from build123d import *

# Parameters (mm, degrees)
ESQUISSE1_R        = 6.75
ESQUISSE1_R_2      = 172
BOSS_EXTRU_1_DEPTH = 10


with BuildPart() as part:
    # Esquisse1 → Boss.-Extru.1 (new body)
    with BuildSketch(Plane.XY):
        with BuildLine():
            Line((220, -35), (220, -297.575677416))
            Line((220, -297.575677416), (190, -380))
            Line((190, -380), (165, -380))
            Line((165, -380), (165, -180))
            Line((165, -180), (125, -180))
            Line((125, -180), (125, -330))
            Line((125, -330), (-125, -330))
            Line((-125, -330), (-125, -180))
            Line((-125, -180), (-165, -180))
            Line((-165, -180), (-165, -380))
            Line((-165, -380), (-190, -380))
            Line((-190, -380), (-220, -297.575677416))
            Line((-220, -297.575677416), (-220, -35))
            Line((-220, -35), (-240, -35))
            Line((-240, -35), (-250, -25))
            Line((-250, -25), (-250, -20))
            Line((-250, -20), (-210, -20))
            Line((-210, -20), (-210, 20))
            Line((-210, 20), (-250, 20))
            Line((-250, 20), (-250, 25))
            Line((-250, 25), (-240, 35))
            Line((-240, 35), (-217.19806629, 35))
            ThreePointArc((-217.19806629, 35), (-155.563491861, 155.563491861), (-35, 217.19806629))
            Line((-35, 217.19806629), (-35, 240))
            Line((-35, 240), (-25, 250))
            Line((-25, 250), (-20, 250))
            Line((-20, 250), (-20, 210))
            Line((-20, 210), (20, 210))
            Line((20, 210), (20, 250))
            Line((20, 250), (25, 250))
            Line((25, 250), (35, 240))
            Line((35, 240), (35, 217.19806629))
            ThreePointArc((35, 217.19806629), (155.563491861, 155.563491861), (217.19806629, 35))
            Line((217.19806629, 35), (240, 35))
            Line((240, 35), (250, 25))
            Line((250, 25), (250, 20))
            Line((250, 20), (210, 20))
            Line((210, 20), (210, -20))
            Line((210, -20), (250, -20))
            Line((250, -20), (250, -25))
            Line((250, -25), (240, -35))
            Line((240, -35), (220, -35))
        make_face()
        with Locations((0, 195)):
            Circle(ESQUISSE1_R, mode=Mode.SUBTRACT)
        Circle(ESQUISSE1_R_2, mode=Mode.SUBTRACT)
        with Locations((52.610370376, 187.768871033)):
            Circle(ESQUISSE1_R, mode=Mode.SUBTRACT)
        with Locations((101.318870257, 166.611783887)):
            Circle(ESQUISSE1_R, mode=Mode.SUBTRACT)
        with Locations((142.513013034, 133.097862928)):
            Circle(ESQUISSE1_R, mode=Mode.SUBTRACT)
        with Locations((173.137617588, 89.712682358)):
            Circle(ESQUISSE1_R, mode=Mode.SUBTRACT)
        with Locations((190.921397098, 39.673922545)):
            Circle(ESQUISSE1_R, mode=Mode.SUBTRACT)
        with Locations((194.545409992, -13.307270606)):
            Circle(ESQUISSE1_R, mode=Mode.SUBTRACT)
        with Locations((183.740879813, -65.301524373)):
            Circle(ESQUISSE1_R, mode=Mode.SUBTRACT)
        with Locations((159.309129137, -112.452662812)):
            Circle(ESQUISSE1_R, mode=Mode.SUBTRACT)
        with Locations((123.062149144, -151.263701687)):
            Circle(ESQUISSE1_R, mode=Mode.SUBTRACT)
        with Locations((77.68821252, -178.856203794)):
            Circle(ESQUISSE1_R, mode=Mode.SUBTRACT)
        with Locations((26.552496574, -193.183759477)):
            Circle(ESQUISSE1_R, mode=Mode.SUBTRACT)
        with Locations((-26.552496574, -193.183759477)):
            Circle(ESQUISSE1_R, mode=Mode.SUBTRACT)
        with Locations((-77.68821252, -178.856203794)):
            Circle(ESQUISSE1_R, mode=Mode.SUBTRACT)
        with Locations((-123.062149144, -151.263701687)):
            Circle(ESQUISSE1_R, mode=Mode.SUBTRACT)
        with Locations((-159.309129137, -112.452662812)):
            Circle(ESQUISSE1_R, mode=Mode.SUBTRACT)
        with Locations((-183.740879813, -65.301524373)):
            Circle(ESQUISSE1_R, mode=Mode.SUBTRACT)
        with Locations((-194.545409992, -13.307270606)):
            Circle(ESQUISSE1_R, mode=Mode.SUBTRACT)
        with Locations((-190.921397098, 39.673922545)):
            Circle(ESQUISSE1_R, mode=Mode.SUBTRACT)
        with Locations((-173.137617588, 89.712682358)):
            Circle(ESQUISSE1_R, mode=Mode.SUBTRACT)
        with Locations((-142.513013034, 133.097862928)):
            Circle(ESQUISSE1_R, mode=Mode.SUBTRACT)
        with Locations((-101.318870257, 166.611783887)):
            Circle(ESQUISSE1_R, mode=Mode.SUBTRACT)
        with Locations((-52.610370376, 187.768871033)):
            Circle(ESQUISSE1_R, mode=Mode.SUBTRACT)
    extrude(amount=BOSS_EXTRU_1_DEPTH)


solid = part.part
Could you check a few things on this model? Use its own coordinates, in mm. Give positions to 0.01 mm unless a question says otherwise; leave off trailing zeros. Write each loop counter-clockwise with the first axis right and the second up, starting at its lowest first coordinate (ties: lowest second). Pieces come first, ordered by that corner, then holes. Notation, with made-up numbers: (22.25, 87) -> (60.25, 87) arc R22 cw to (60.25, 94) -> close; hole circle Ø3 at (19.25, 72). An arc over 180 degrees is marked (long way). Write each question's results on one line, items separated by ' | '. Start each with the question number.
Q1. I'm going to push flat-ended pins straight in: pin 1 Ø12 at (x, y) = (-77.69, -178.86) entering from -Z; pin 2 Ø3 at (y, z) = (237, 3) entering from +X; pin 3 Ø3 at (y, z) = (54, 8) entering from -X; pin 4 Ø2 at (x, z) = (-42, 6.5) entering from -Y. Where does each tip first touch, or does it pass through?
Q2. Suppose I cut it at B-B, the plane x = 0. List the corners of the cut face in (y, z) for me, and give its area (4 significant figures).
Q3. I need wall thicknesses on probe 1 along Y at (x, z) = (-1, 3); probe 2 along X at (y, z) = (-293, 3.25); probe 3 along Y at (x, z) = (107.5, 8). Which ranges of each line are inside material? Lowest first, please.
Q4. Suppose I cut it at A-A, the plane y = 0. List the corners of the cut face in (x, z) for me.
Q5. Suppose I cut it at C-C, the plane y = 103. List the corners of the cut face in (x, z) for me.
Q6. We'd pull the mould along X, two halves only. Please class faces 1 (the face through (-204.79, -339.36, 4.93)), 2 (the face through (-57.585, 192.331, 4.93)), 3 (the face through (38, -180, 0)), 4 (the face through (-180.11, -59.61, 4.93)): +X half, -X half, draft (parallel to the pull), parting line (faces both ways), or undercut.
Q7. Suppose I cut it at D-D, the plane z = 3.75. State how many separate pieces and enclosed holes the cut face has, and give its area (3 significant figures).
Outcome:
1) pin 1: through | pin 2: x = 35 | pin 3: x = -213.64 | pin 4: y = -330
2) outline: (-330, 0) -> (-172, 0) -> (-172, 10) -> (-330, 10) -> close; (172, 0) -> (188.25, 0) -> (188.25, 10) -> (172, 10) -> close; (201.75, 0) -> (210, 0) -> (210, 10) -> (201.75, 10) -> close | area: 1,825 mm2
3) probe 1: -330 to -172, 172 to 188.32, 201.68 to 210 | probe 2: -220 to -165, -125 to 125, 165 to 220 | probe 3: -330 to -134.27, 134.27 to 163.9, 169.32 to 191.95
4) outline: (-210, 0) -> (-172, 0) -> (-172, 10) -> (-210, 10) -> close; (172, 0) -> (210, 0) -> (210, 10) -> (172, 10) -> close
5) outline: (-194.4, 0) -> (-137.75, 0) -> (-137.75, 10) -> (-194.4, 10) -> close; (137.75, 0) -> (194.4, 0) -> (194.4, 10) -> (137.75, 10) -> close
6) face 1: -X half | face 2: undercut | face 3: draft | face 4: undercut
7) separate pieces: 1 | enclosed holes: 24 | area: 117,000 mm2
